Model file for the job. Use its own axes, mm. Face numbers are marked on the shaded views. Round coordinates to 2 decimals unless told otherwise and drop trailing zeros. Write each loop counter-clockwise with the first axis right and the second up, starting at its lowest first coordinate (ties: lowest second). Pieces come first, ordered by that corner, then holes. Notation, with made-up numbers: (0.25, 30.25) - (28.25, 30.25) arc R4 cw to (28.25, 36.25) - close; hole circle Ø8 at (46, 35). An arc over 180 degrees is marked (long way). One line per item, written item: value.
Autodesk Inventor part; units mm, degrees
ref_plane "YZ Plane" through (0, 0, 0) normal (1, 0, 0) x (0, 1, 0)
ref_plane "XZ Plane" through (0, 0, 0) normal (0, 1, 0) x (-1, 0, 0)
ref_plane "XY Plane" through (0, 0, 0) normal (0, 0, 1) x (1, 0, 0)
sketch "Эскиз1" plane through (0, 0, 0) normal (0, 0, 1) x (1, 0, 0)
  circle A0 centre (0, 0) radius 60
  circle A1 centre (0, 0) radius 55
  dimension "d0" = 120
  dimension "d1" = 110
extrude "Выдавливание1" add sketch "Эскиз1" along normal blind 51
sketch "Эскиз2" plane through (0, 0, 51) normal (0, 0, 1) x (1, 0, 0)
  circle A0 centre (0, 0) radius 60
  circle A1 centre (0, 0) radius 65
extrude "Выдавливание2" add sketch "Эскиз2" against normal blind 4
sketch "Эскиз3" plane through (0, 0, 51) normal (0, 0, 1) x (1, 0, 0)
  circle A0 centre (0, 0) radius 55
  line L0 (0, 55) -> (0, 62.5)
  dimension "d6" = 7.5
hole "Отверстие1" at (0, 62.5, 51) direction (0, 0, -1) diameter 4 depth 15 tip angle 118
mirror "Зеркальное отражение1" about plane through (0, 0, 0) normal (0, 1, 0) of "Отверстие1"
properties part number "Втулка под палец" material "Бронза, литейная"
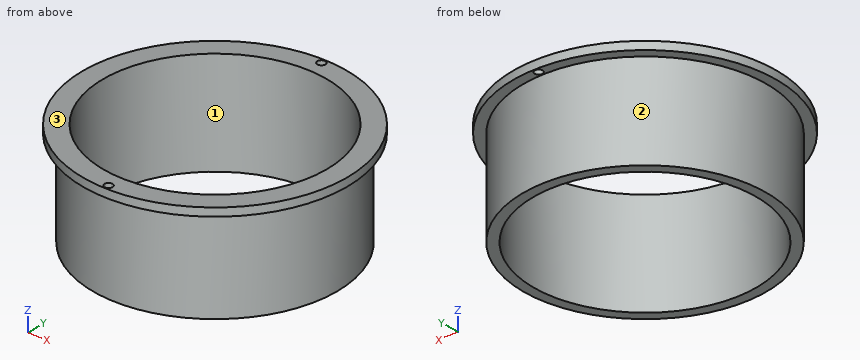
1. Drop flat-ended pins along their axis: pin 1 (1.5 mm diameter, centred on x = 28, z = 11.5, fed in from -Y) (3 decimals); pin 2 (1 mm diameter, centred on y = 50, z = 22.5, fed in from -X); pin 3 (12 mm diameter, centred on y = -9, z = 5, fed in from -X); pin 4 (10 mm diameter, centred on x = -24, y = 39.5, fed in from +Z). Give the stop position or say it passes through.
Report:
pin 1: y = -53.455
pin 2: x = -33.91
pin 3: x = -59.92
pin 4: through
2. Band-saw the part on D-D on z = 40.5. Write the cut outline in (x, y).
Report:
outline: circle Ø120 at (0, 0); hole circle Ø110 at (0, 0)
3. Mould opens along Y. For the marked faces 1, 2 and 3 say: released by +Y, released by -Y, zero draft, split by the parting line, or undercut.
Report:
face 1: undercut
face 2: split by the parting line
face 3: zero draft
4. Band-saw the part on C-C on x = -30.5. Write the cut outline in (y, z).
Report:
outline: (-57.4, 47) - (-51.67, 47) - (-51.67, 0) - (-45.77, 0) - (-45.77, 51) - (-57.4, 51) - close; (45.77, 0) - (51.67, 0) - (51.67, 47) - (57.4, 47) - (57.4, 51) - (45.77, 51) - close
5. Wall check: probe 1 along Y at (x, z) = (0, 49); probe 2 along Y at (x, z) = (0, 28); probe 3 along X at (y, z) = (36.5, 22). Give the ranges that are in metal, low to high. Write a range as [from, to].
Report:
probe 1: [-65, -64.5], [-60.5, -55], [55, 60.5], [64.5, 65]
probe 2: [-60, -55], [55, 60]
probe 3: [-47.62, -41.14], [41.14, 47.62]
6. Band-saw the part on B-B on x = 0. Write the cut outline in (y, z).
Report:
outline: (-65, 47) - (-64.5, 47) - (-64.5, 51) - (-65, 51) - close; (-60.5, 47) - (-60, 47) - (-60, 0) - (-55, 0) - (-55, 51) - (-60.5, 51) - close; (55, 0) - (60, 0) - (60, 47) - (60.5, 47) - (60.5, 51) - (55, 51) - close; (64.5, 47) - (65, 47) - (65, 51) - (64.5, 51) - close
7. Band-saw the part on A-A on y = 0. Write the cut outline in (x, z).
Report:
outline: (-65, 47) - (-60, 47) - (-60, 0) - (-55, 0) - (-55, 51) - (-65, 51) - close; (55, 0) - (60, 0) - (60, 47) - (65, 47) - (65, 51) - (55, 51) - close
